from build123d import *

# Parameters (mm, degrees)
SKETCH1_R               = 87.5
BOSS_EXTRUDE1_DEPTH     = 60
SKETCH2_R               = 85
CUT_EXTRUDE1_DEPTH      = 55
CUT_EXTRUDE2_REACH      = 137.416
SKETCH3_R               = 41.5
CUT_EXTRUDE3_REACH      = 206.649
CUT_EXTRUDE3_END_RADIUS = 85
SKETCH4_W               = 25
SKETCH4_H               = 20
CUT_EXTRUDE5_REACH      = 206.649
CUT_EXTRUDE5_END_RADIUS = 85
SKETCH5_W               = 6.2
SKETCH5_H               = 6.2
SKETCH5_H_2             = 6.393620859


with BuildPart() as part:
    # Sketch1 → Boss-Extrude1 (new body)
    with BuildSketch(Plane(origin=(0, 0, 0), x_dir=(1, 0, 0), z_dir=(0, 1, 0))):
        with Locations(Location((0, 0, 0), (0, 0, 270))):
            Circle(SKETCH1_R)
    extrude(amount=BOSS_EXTRUDE1_DEPTH)

    # Sketch2 → Cut-Extrude1 (cut)
    with BuildSketch(Plane.XZ):
        with Locations(Location((0, 0, 0), (0, 0, 270))):
            Circle(SKETCH2_R)
    extrude(amount=-CUT_EXTRUDE1_DEPTH, mode=Mode.SUBTRACT)

    # Sketch3 → Cut-Extrude2 (cut, up to next)
    with BuildSketch(Plane.XZ.offset(-55), mode=Mode.PRIVATE) as cut_extrude2_sk1:
        with Locations(Location((0, 0, 0), (0, 0, 270))):
            Circle(SKETCH3_R)
    cut_extrude2_tool1 = extrude(cut_extrude2_sk1.sketch, amount=-CUT_EXTRUDE2_REACH, mode=Mode.PRIVATE) & part.part
    add(cut_extrude2_tool1.solids().sort_by_distance((0, 55, 0))[0], mode=Mode.SUBTRACT)

    # Cut-Extrude3: up to this cylinder (the profile starts outside it)
    cut_extrude3_end = Plane(origin=(0, 10, 0), z_dir=(0, -1, 0)) * Cylinder(CUT_EXTRUDE3_END_RADIUS, 584.298, mode=Mode.PRIVATE)
    # Sketch4 → Cut-Extrude3 (cut, up to the surface)
    with BuildSketch(Plane.XY.offset(87.5), mode=Mode.PRIVATE) as cut_extrude3_sk1:
        with Locations((0, 10)):
            Rectangle(SKETCH4_W, SKETCH4_H)
    cut_extrude3_tool1 = extrude(cut_extrude3_sk1.sketch, amount=-CUT_EXTRUDE3_REACH, mode=Mode.PRIVATE) - cut_extrude3_end
    add(cut_extrude3_tool1.solids().sort_by_distance((0, 10, 87.5))[0], mode=Mode.SUBTRACT)

    # Cut-Extrude5: up to this cylinder (the profile starts outside it)
    cut_extrude5_end = Plane(origin=(0, 43.356907, 0), z_dir=(0, -1, 0)) * Cylinder(CUT_EXTRUDE5_END_RADIUS, 584.39481, mode=Mode.PRIVATE)
    # Sketch5 → Cut-Extrude5 (cut, up to the surface)
    with BuildSketch(Plane.XY.offset(-87.5), mode=Mode.PRIVATE) as cut_extrude5_sk1:
        with Locations((10, 43.405312256)):
            Rectangle(SKETCH5_W, SKETCH5_H)
    cut_extrude5_tool1 = extrude(cut_extrude5_sk1.sketch, amount=CUT_EXTRUDE5_REACH, mode=Mode.PRIVATE) - cut_extrude5_end
    add(cut_extrude5_tool1.solids().sort_by_distance((10, 43.405312, -87.5))[0], mode=Mode.SUBTRACT)
    # Sketch5 → Cut-Extrude5 (cut, up to the surface)
    with BuildSketch(Plane.XY.offset(-87.5), mode=Mode.PRIVATE) as cut_extrude5_sk2:
        with Locations((-10, 43.308501827)):
            Rectangle(SKETCH5_W, SKETCH5_H_2)
    cut_extrude5_tool2 = extrude(cut_extrude5_sk2.sketch, amount=CUT_EXTRUDE5_REACH, mode=Mode.PRIVATE) - cut_extrude5_end
    add(cut_extrude5_tool2.solids().sort_by_distance((-10, 43.308502, -87.5))[0], mode=Mode.SUBTRACT)


solid = part.part
Here's how the part is built. I have some questions about the finished solid (model axes, mm). A direction names the side the tool comes from. Round coordinates to 2 decimals unless told otherwise and drop trailing zeros. Order: outer loops, then holes, each group sorted by start corner. A loop starts at its lowest first (then second) coordinate and runs counter-clockwise, first axis right, second up. Notation, with made-up numbers: M -21,54 L -12,54 A28 cw -12,92 Z; hole C -38,-29 d1. An arc over 180 degrees is marked long. Return JSON: item names as keys, results as strings. Group by question number.
1. If we section it at C-C on y = 25: List the corners of the cut face in (x, z) for me, then the cut area to 3 significant figures.
2. If we section it at A-A on z = 0: List the corners of the cut face in (x, y) for me, then the cut area to 3 significant figures.
3. If we section it at D-D on x = -54: List the corners of the cut face in (y, z) for me, then the cut area to 3 significant figures.
4. If we section it at B-B on x = 0: List the corners of the cut face in (y, z) for me, then the cut area to 3 significant figures.
5. If we mould it in two halves opening along X, with no side actions, what happens to faces 3 (the face through (12.465, 57.465, -39.584)), 4 (the face through (86.755, 29.58, -11.391)), 5 (the face through (-38, 0, 77))? For each: pulls with the +X half, pulls with the -X half, needs draft (parallel to the pull), parting line crosses it, or undercut.
6. Please list where these lines run through material, in increasing order: probe 1 along X at (y, z) = (24, 0); probe 2 along X at (y, z) = (57.1, 0); probe 3 along Y at (x, z) = (-40.5, -12).
7. I'm going to push flat-ended pins straight in: pin 1 Ø3 at (x, y) = (23.5, 27.5) entering from +Z; pin 2 Ø1.5 at (x, y) = (42.5, 51.5) entering from -Z; pin 3 Ø4 at (x, y) = (-68, 20.5) entering from +Z. Where does each tip first touch, or does it pass through?
8. On a 3-axis mill with a long thin cutter (end or side, diameter ignored), from which of +Z, -Z, +X, -X, +Y, -Y can I reach the whole of each face in a straight line? I mean faces 1 (the face through (-37, 55, 20)), 2 (the face through (-18, 60, 38)). Say none if no direction works.
Reply:
{
 "1": {"outline": "C 0,0 d175; hole C 0,0 d170", "area": "1,350 mm^2"},
 "2": {"outline": "M -87.5,0 L -85,0 L -85,55 L -41.5,55 L -41.5,60 L -87.5,60 Z; M 41.5,55 L 85,55 L 85,0 L 87.5,0 L 87.5,60 L 41.5,60 Z", "area": "735 mm^2"},
 "3": {"outline": "M 0,-68.85 L 60,-68.85 L 60,68.85 L 0,68.85 L 0,65.64 L 55,65.64 L 55,-65.64 L 0,-65.64 Z", "area": "1,040 mm^2"},
 "4": {"outline": "M 0,-87.5 L 60,-87.5 L 60,-41.5 L 55,-41.5 L 55,-85 L 0,-85 Z; M 20,85 L 55,85 L 55,41.5 L 60,41.5 L 60,87.5 L 20,87.5 Z", "area": "685 mm^2"},
 "5": {"face 3": "undercut", "face 4": "parting line crosses it", "face 5": "needs draft"},
 "6": {"probe 1": "-87.5 to -85, 85 to 87.5", "probe 2": "-87.5 to -41.5, 41.5 to 87.5", "probe 3": "55 to 60"},
 "7": {"pin 1": "z = 84.69", "pin 2": "z = -76.9", "pin 3": "z = 57.45"},
 "8": {"face 1": "-Y", "face 2": "+Z, -Z, +X, -X, +Y"}
}
